Check sheet for the drawn part. Datum: minimum x, y, z corner. Units: mm. Give positions to 0.01 mm unless a question says otherwise; leave off trailing zeros. Write each loop counter-clockwise with the first axis right and the second up, starting at its lowest first coordinate (ties: lowest second). Pieces come first, ordered by that corner, then holes. Notation, with made-up numbers: (0.25, 3) -> (22.25, 3) arc R28 cw to (22.25, 21) -> close; hole circle Ø7 at (30, 17.5). An arc over 180 degrees is marked (long way). Write item = value, one per line. Start each with the question number.
1. Cross-section at A-A, the plane x = 5. Record the cut outline in (y, z), plus the area to 3 significant figures.
2. Thickness scan on line 1 along Y through (x, z) = (5, 1.25); line 2 along X through (y, z) = (136, 0.75); line 3 along Y through (x, z) = (37, 2.9). Record the ranges inside material, lowest first.
3. Depth check by flat-ended pin: P1, Ø5, axis at x = 35, y = 110, coming from the -Z side. Enter the tip coordinate at first touch or a pass-through.
4. Cross-section at B-B, the plane y = 41. Record the cut outline in (x, z), plus the area to 3 significant figures.
5. Cross-section at C-C, the plane z = 0.8. State how many separate pieces and enclosed holes the cut face has, plus the area to 3 significant figures.
6. Cross-section at D-D, the plane y = 150. Record the cut outline in (x, z).
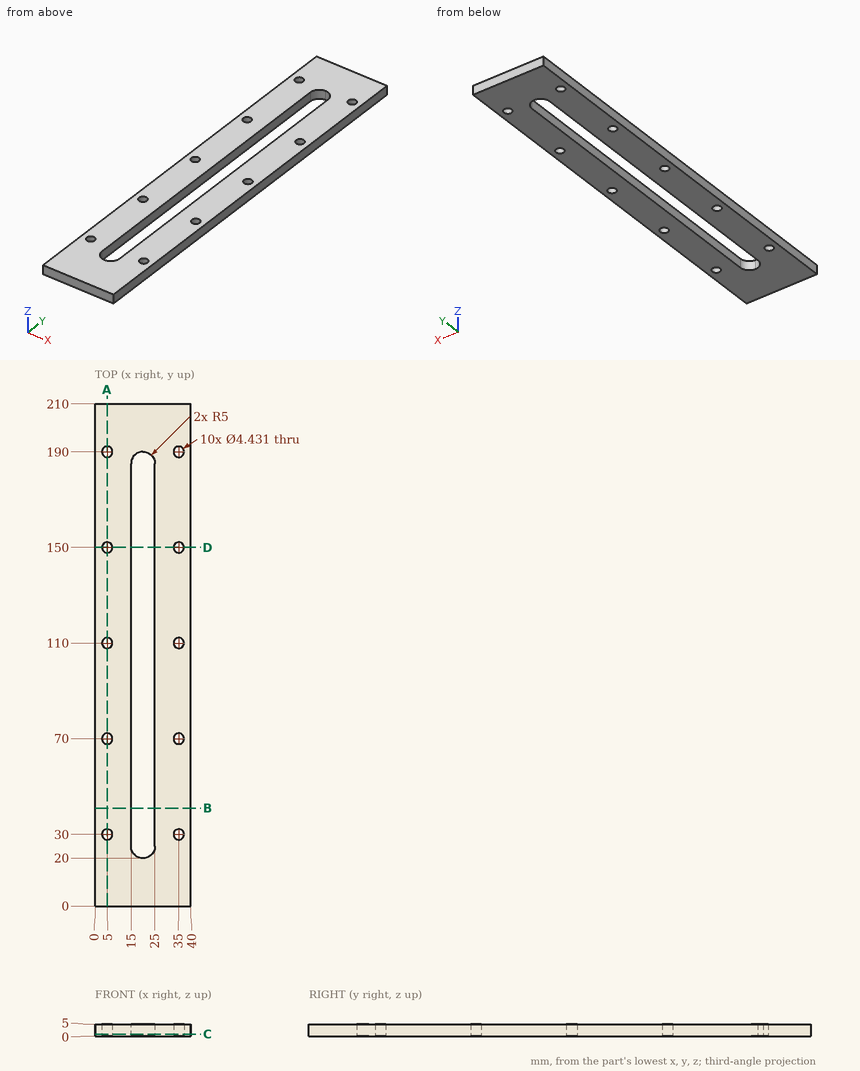
Answers:
q1.outline = (0, 0) -> (27.78, 0) -> (27.78, 5) -> (0, 5) -> close; (32.22, 0) -> (67.78, 0) -> (67.78, 5) -> (32.22, 5) -> close; (72.22, 0) -> (107.78, 0) -> (107.78, 5) -> (72.22, 5) -> close; (112.22, 0) -> (147.78, 0) -> (147.78, 5) -> (112.22, 5) -> close; (152.22, 0) -> (187.78, 0) -> (187.78, 5) -> (152.22, 5) -> close; (192.22, 0) -> (210, 0) -> (210, 5) -> (192.22, 5) -> close
q1.area = 939 mm^2
q2.line_1 = 0 to 27.78, 32.22 to 67.78, 72.22 to 107.78, 112.22 to 147.78, 152.22 to 187.78, 192.22 to 210
q2.line_2 = 0 to 15, 25 to 40
q2.line_3 = 0 to 29.05, 30.95 to 69.05, 70.95 to 109.05, 110.95 to 149.05, 150.95 to 189.05, 190.95 to 210
q3.P1 = 0
q4.outline = (0, 0) -> (15, 0) -> (15, 5) -> (0, 5) -> close; (25, 0) -> (40, 0) -> (40, 5) -> (25, 5) -> close
q4.area = 150 mm^2
q5.separate_pieces = 1
q5.enclosed_holes = 11
q5.area = 6,570 mm^2
q6.outline = (0, 0) -> (2.78, 0) -> (2.78, 5) -> (0, 5) -> close; (7.22, 0) -> (15, 0) -> (15, 5) -> (7.22, 5) -> close; (25, 0) -> (32.78, 0) -> (32.78, 5) -> (25, 5) -> close; (37.22, 0) -> (40, 0) -> (40, 5) -> (37.22, 5) -> close
